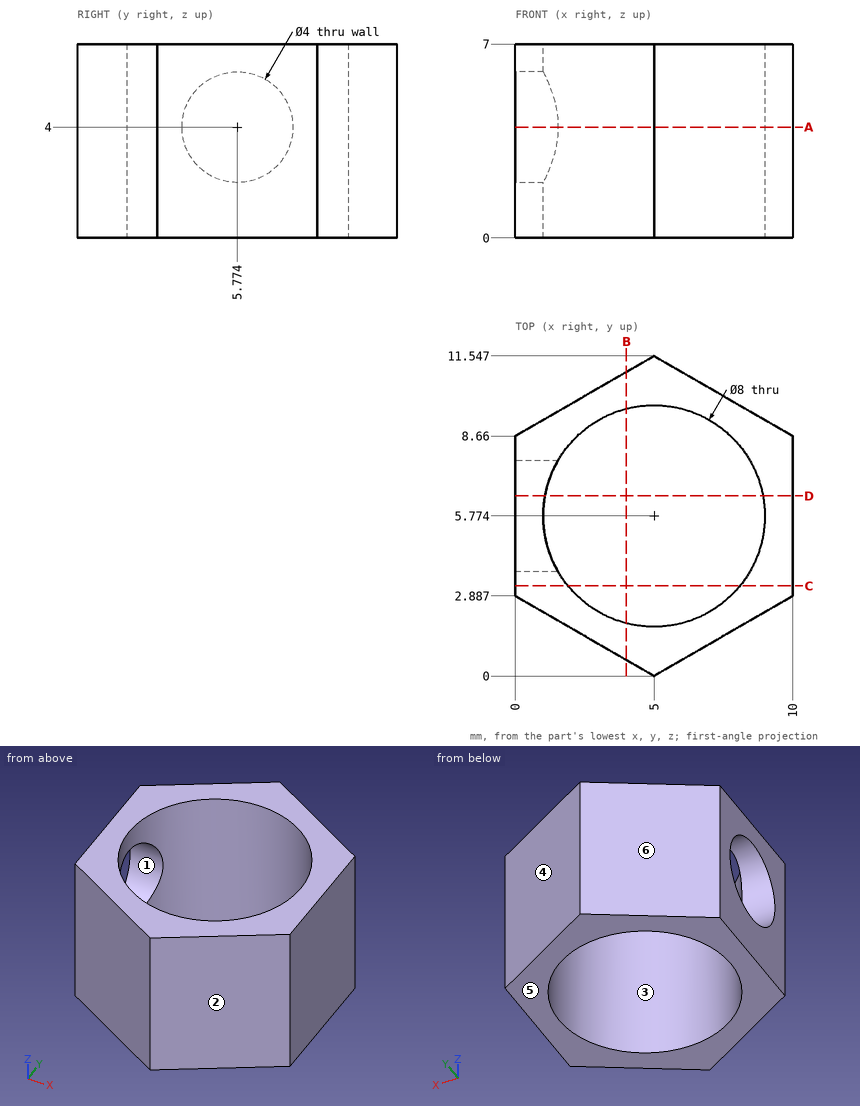
Check sheet for the drawn part. Datum: minimum x, y, z corner. Units: mm. A direction names the side the tool comes from. Coordinates: 2 decimals unless noted, no trailing zeros. Order: outer loops, then holes, each group sorted by start corner. A loop starts at its lowest first (then second) coordinate and runs counter-clockwise, first axis right, second up. Notation, with made-up numbers: M -10,30 L 49,30 A21 ccw 49,58 Z; hole C 50.25,-39 d5. An arc over 180 degrees is marked long. One line per item, written item: value. Start each with the question number.
Item 1: Access from +Z, -Z, +X, -X, +Y, -Y to the whole of each face (thin tool, end or side, straight path). Record for the marked faces 1 and 2.
Item 2: Sectioned sample at B-B (x = 4). Enter the section's corners in (y, z).
Item 3: Scan lines: probe 1 along Y at (x, z) = (2, 1.75) (1 decimal); probe 2 along X at (y, z) = (8.5, 3) (1 decimal); probe 3 along Z at (x, y) = (1.25, 4) (1 decimal). Record each from-to range of solid material in increasing order.
Item 4: Mould release check, pull along X, two halves, no side actions. Record for the marked faces 3, 4, 5 and 6: released by +X, released by -X, zero draft, split by the parting line, or undercut.
Item 5: Sectioned sample at D-D (y = 6.5). Enter the section's corners in (x, z).
Item 6: Sectioned sample at C-C (y = 3.25). Enter the section's corners in (x, z).
Item 7: Gauge pin test, flat ends, axial feed: pin 1 (1.5 mm diameter, centred on x = 5.5, z = 5.5, fed in from -Y); pin 2 (2 mm diameter, centred on y = 10, z = 2, fed in from -X). Record the tip position at first contact, or that the pin passes through.
Item 8: Sectioned sample at A-A (z = 4). Enter the section's corners in (x, y) (1 decimal).
Conclusion:
1. face 1: -X
1. face 2: +Z, -Z, +X, -Y
2. outline: M 0.58,0 L 1.9,0 L 1.9,7 L 0.58,7 Z; M 9.65,0 L 10.97,0 L 10.97,7 L 9.65,7 Z
3. probe 1: y = 1.7 to 3.1, 8.4 to 9.8
3. probe 2: x = 0 to 2.1, 7.9 to 10
3. probe 3: z = 0 to 3.1, 4.9 to 7
4. face 3: undercut
4. face 4: released by +X
4. face 5: zero draft
4. face 6: released by -X
5. outline: M 0,0 L 1.07,0 L 1.07,2.14 L 0,2.14 Z; M 0,5.86 L 1.07,5.86 L 1.07,7 L 0,7 Z; M 8.93,0 L 10,0 L 10,7 L 8.93,7 Z
6. outline: M 0,0 L 1.9,0 L 1.9,7 L 0,7 Z; M 8.1,0 L 10,0 L 10,7 L 8.1,7 Z
7. pin 1: stops at y = 0
7. pin 2: stops at x = 0.59
8. outline: M 0,2.9 L 5,0 L 10,2.9 L 10,8.7 L 5,11.5 L 0,8.7 L 0,7.8 L 1.5,7.8 A4 cw long 1.5,3.8 L 0,3.8 Z
